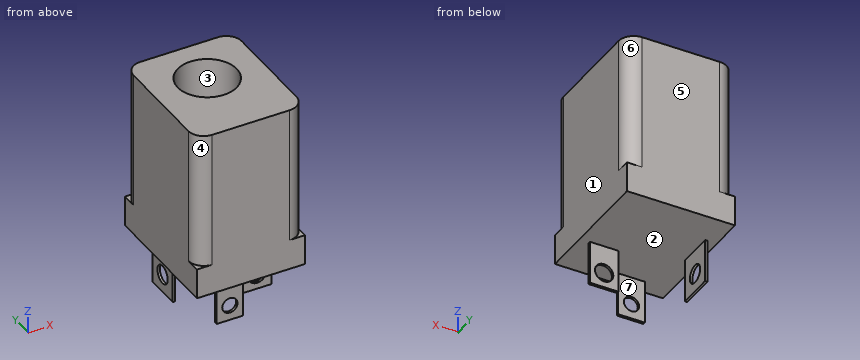
```python
from build123d import *

# Parameters (mm, degrees)
BOSS_EXTRUDE1_DEPTH = 13.9954
SKETCH2_R           = 2.453758577
CUT_EXTRUDE1_DEPTH  = 9.2456
SKETCH3_W           = 8.9916
SKETCH3_H           = 10.6934
BOSS_EXTRUDE2_DEPTH = 2.54
SKETCH4_W           = 0.2032
SKETCH4_H           = 2.9972
SKETCH4_W_2         = 2.2098
SKETCH4_H_2         = 0.2032
SKETCH4_W_3         = 2.3876
BOSS_EXTRUDE3_DEPTH = 3.6068
CUT_EXTRUDE2_REACH  = 24.099
SKETCH5_R           = 0.762
CUT_EXTRUDE3_REACH  = 22.96
SKETCH6_R           = 0.762
CUT_EXTRUDE4_REACH  = 23.926
SKETCH7_R           = 0.635


with BuildPart() as part:
    # Sketch1 → Boss-Extrude1 (new body)
    with BuildSketch(Plane.XY):
        with BuildLine():
            Line((1.27, 0), (7.7216, 0))
            ThreePointArc((7.7216, 0), (8.619625612, 0.371974388), (8.9916, 1.27))
            Line((8.9916, 1.27), (8.9916, 9.4234))
            ThreePointArc((8.9916, 9.4234), (8.619625612, 10.321425612), (7.7216, 10.6934))
            Line((7.7216, 10.6934), (1.27, 10.6934))
            ThreePointArc((1.27, 10.6934), (0.371974388, 10.321425612), (0, 9.4234))
            Line((0, 9.4234), (0, 1.27))
            ThreePointArc((0, 1.27), (0.371974388, 0.371974388), (1.27, 0))
        make_face()
    extrude(amount=-BOSS_EXTRUDE1_DEPTH)

    # Sketch2 → Cut-Extrude1 (cut)
    with BuildSketch(Plane.XY):
        with Locations((4.4958, 6.5024)):
            Circle(SKETCH2_R)
    extrude(amount=-CUT_EXTRUDE1_DEPTH, mode=Mode.SUBTRACT)

    # Sketch3 → Boss-Extrude2 (add)
    with BuildSketch(Plane(origin=(0, 0, -13.9954), x_dir=(-1, 0, 0), z_dir=(0, 0, -1))):
        with Locations((-4.4958, 5.3467)):
            Rectangle(SKETCH3_W, SKETCH3_H)
    extrude(amount=-BOSS_EXTRUDE2_DEPTH)

    # Sketch4 → Boss-Extrude3 (add)
    with BuildSketch(Plane(origin=(0, 0, -13.9954), x_dir=(-1, 0, 0), z_dir=(0, 0, -1))):
        with Locations((-0.87884, 6.5024)):
            Rectangle(SKETCH4_W, SKETCH4_H)
        with Locations((-3.302, 1.10236)):
            Rectangle(SKETCH4_W_2, SKETCH4_H_2)
        with Locations((-6.985, 3.61696)):
            Rectangle(SKETCH4_W_3, SKETCH4_H_2)
    extrude(amount=BOSS_EXTRUDE3_DEPTH)

    # Sketch5 → Cut-Extrude2 (cut, up to next)
    with BuildSketch(Plane(origin=(0.98044, 0, 0), x_dir=(0, 0, -1), z_dir=(1, 0, 0)), mode=Mode.PRIVATE) as cut_extrude2_sk1:
        with Locations((16.0782, 6.5024)):
            Circle(SKETCH5_R)
    cut_extrude2_tool1 = extrude(cut_extrude2_sk1.sketch, amount=-CUT_EXTRUDE2_REACH, mode=Mode.PRIVATE) & part.part
    add(cut_extrude2_tool1.solids().sort_by_distance((0.98044, 6.5024, -16.0782))[0], mode=Mode.SUBTRACT)

    # Sketch6 → Cut-Extrude3 (cut, up to next)
    with BuildSketch(Plane(origin=(0, 3.71856, 0), x_dir=(1, 0, 0), z_dir=(0, 1, 0)), mode=Mode.PRIVATE) as cut_extrude3_sk1:
        with Locations(Location((6.985, 16.3322, 0), (0, 0, 180))):
            Circle(SKETCH6_R)
    cut_extrude3_tool1 = extrude(cut_extrude3_sk1.sketch, amount=-CUT_EXTRUDE3_REACH, mode=Mode.PRIVATE) & part.part
    add(cut_extrude3_tool1.solids().sort_by_distance((6.985, 3.71856, -16.3322))[0], mode=Mode.SUBTRACT)

    # Sketch7 → Cut-Extrude4 (cut, up to next)
    with BuildSketch(Plane(origin=(0, 1.20396, 0), x_dir=(1, 0, 0), z_dir=(0, 1, 0)), mode=Mode.PRIVATE) as cut_extrude4_sk1:
        with Locations(Location((3.302, 16.3322, 0), (0, 0, 180))):
            Circle(SKETCH7_R)
    cut_extrude4_tool1 = extrude(cut_extrude4_sk1.sketch, amount=-CUT_EXTRUDE4_REACH, mode=Mode.PRIVATE) & part.part
    add(cut_extrude4_tool1.solids().sort_by_distance((3.302, 1.20396, -16.3322))[0], mode=Mode.SUBTRACT)


solid = part.part
```
Part model, mm, in its own coordinate system. Face numbers are marked on the shaded views. A direction names the side the tool comes from. Round coordinates to 2 decimals unless told otherwise and drop trailing zeros. Order: outer loops, then holes, each group sorted by start corner. A loop starts at its lowest first (then second) coordinate and runs counter-clockwise, first axis right, second up. Notation, with made-up numbers: M -21,16 L 23,16 A32 ccw 23,45 Z; hole C -33.5,76 d7. An arc over 180 degrees is marked long. Answer in a Markdown table with one row per item. Add a question column.
Q1. Wall check: L1, parallel to Z at x = 0.75, y = 10; L2, parallel to Y at x = 7, z = -15.25; L3, parallel to Z at x = 6, y = 6. Give the ranges that are in metal, low to high. Write a range as from..to.
Q2. 3-axis set-ups, long thin cutter, end or side, ignore diameter. For the marked faces 5, 6 and 7: which of +Z, -Z, +X, -X, +Y, -Y reach the whole face in a straight line?
Q3. Cut at A-A on z = -14.5. Give the cut face in (x, y), and give its area (3 significant figures).
Q4. Cut at B-B on x = 3.75. Give the cut face in (y, z), and give its area (3 significant figures).
Q5. Cut at D-D on z = -7.5. Give the cut face in (x, y).
Q6. Mould opens along X. For the marked faces 1, 2, 3 and 4 say: +X half, -X half, draft (parallel to the pull), parting line (faces both ways), or undercut.
Q7. Cut at C-C on y = 5.5. Give the cut face in (x, z).
Q8. Pin check, flat tips, straight feed: pin 1 (0.9 mm diameter, centred on y = 6.5, z = -15.5, fed in from -X); pin 2 (1.1 mm diameter, centred on x = 3.3, z = -16.33, fed in from -Y); pin 3 (2.5 mm diameter, centred on x = 6.5, z = -15.5, fed in from -Y); pin 4 (1.9 mm diameter, centred on x = 7.5, z = -16.5, fed in from +Y). Stop position of each tip, or through.
Established:
| question | item | result |
|---|---|---|
| 1 | L1 | z = -14..0 |
| 1 | L2 | y = 3.52..3.72 |
| 1 | L3 | z = -14..-9.25 |
| 2 | face 5 | +Z, -Z, +X, -X, +Y |
| 2 | face 6 | +Z, +X, +Y |
| 2 | face 7 | -Z, +X, -X, +Y |
| 3 | outline | M 0.78,5 L 0.98,5 L 0.98,8 L 0.78,8 Z; M 2.2,1 L 4.41,1 L 4.41,1.2 L 2.2,1.2 Z; M 5.79,3.52 L 8.18,3.52 L 8.18,3.72 L 5.79,3.72 Z |
| 3 | area | 1.54 mm2 |
| 4 | outline | M 0,-14 L 1,-14 L 1,-15.88 L 1.2,-15.88 L 1.2,-14 L 10.69,-14 L 10.69,0 L 8.84,0 L 8.84,-9.25 L 4.16,-9.25 L 4.16,0 L 0,0 Z; M 1,-17.6 L 1.2,-17.6 L 1.2,-16.78 L 1,-16.78 Z |
| 4 | area | 107 mm2 |
| 5 | outline | M 0,1.27 A1.27 ccw 1.27,0 L 7.72,0 A1.27 ccw 8.99,1.27 L 8.99,9.42 A1.27 ccw 7.72,10.69 L 1.27,10.69 A1.27 ccw 0,9.42 Z; hole C 4.5,6.5 d4.91 |
| 6 | face 1 | +X half |
| 6 | face 2 | draft |
| 6 | face 3 | undercut |
| 6 | face 4 | -X half |
| 7 | outline | M 0,-14 L 0.78,-14 L 0.78,-17.6 L 0.98,-17.6 L 0.98,-14 L 8.99,-14 L 8.99,0 L 6.74,0 L 6.74,-9.25 L 2.26,-9.25 L 2.26,0 L 0,0 Z |
| 8 | pin 1 | stops at x = 0.78 |
| 8 | pin 2 | passes through |
| 8 | pin 3 | stops at y = 3.52 |
| 8 | pin 4 | stops at y = 3.72 |
